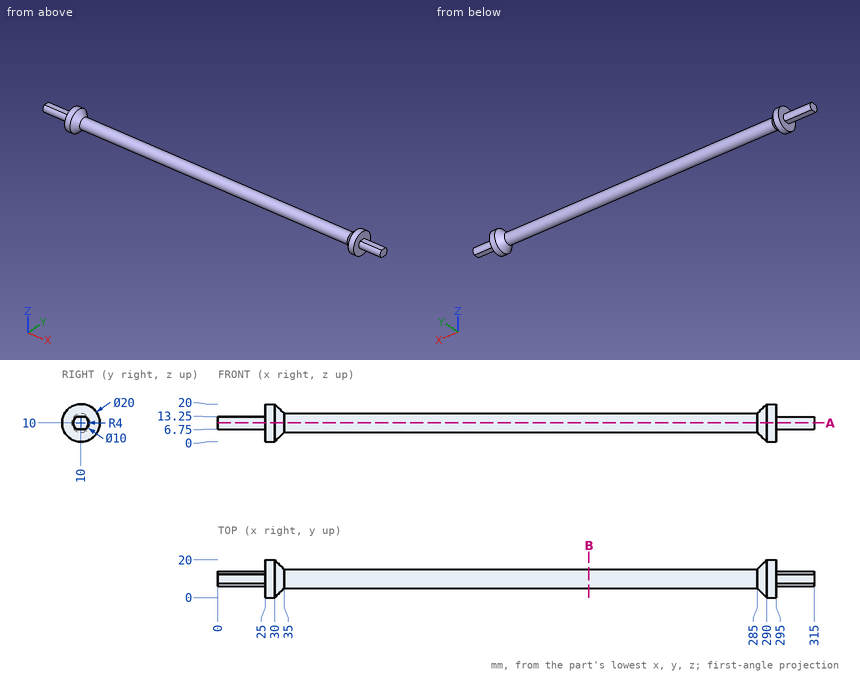
Could you check a few things on this drawing? It's one solid part, dimensions in mm from its lowest x, y, z. Coordinates: 2 decimals unless noted, no trailing zeros. Order: outer loops, then holes, each group sorted by start corner. A loop starts at its lowest first (then second) coordinate and runs counter-clockwise, first axis right, second up. Notation, with made-up numbers: M 20,18 L 46,18 A23 cw 46,37 Z; hole C 24,-26 d4. An arc over 180 degrees is marked long. Use a Markdown table: item, result. Add a question column.
Q1. I'm going to push flat-ended pins straight in: pin 1 (1.5 mm diameter, centred on y = 2.5, z = 13.5, fed in from +X); pin 2 (3 mm diameter, centred on x = 237, z = 10, fed in from -Y); pin 3 (2.5 mm diameter, centred on x = 302, y = 9, fed in from +Z). Where does each tip first touch, or does it pass through?
Q2. I want a section at B-B on x = 196. List the corners of the cut face in (y, z) for me.
Q3. I want a section at A-A on z = 10. List the corners of the cut face in (x, y) for me.
Q4. If I drill on L1, parallel to X at y = 12.75, z = 17.5; L2, parallel to Z at x = 164, y = 13; L3, parallel to X at y = 8.5, z = 4, over which ranges is the centre line in solid material (lowest first)?
Checked values:
| question | item | result |
|---|---|---|
| 1 | pin 1 | x = 295 |
| 1 | pin 2 | y = 5 |
| 1 | pin 3 | z = 13.25 |
| 2 | outline | C 10,10 d10 |
| 3 | outline | M 0,6 L 25,6 L 25,0 L 30,0 L 35,5 L 285,5 L 290,0 L 295,0 L 295,6 L 315,6 L 315,14 L 295,14 L 295,20 L 290,20 L 285,15 L 35,15 L 30,20 L 25,20 L 25,14 L 0,14 Z |
| 4 | L1 | 25 to 32.01, 287.99 to 295 |
| 4 | L2 | 6 to 14 |
| 4 | L3 | 25 to 33.82, 286.18 to 295 |
